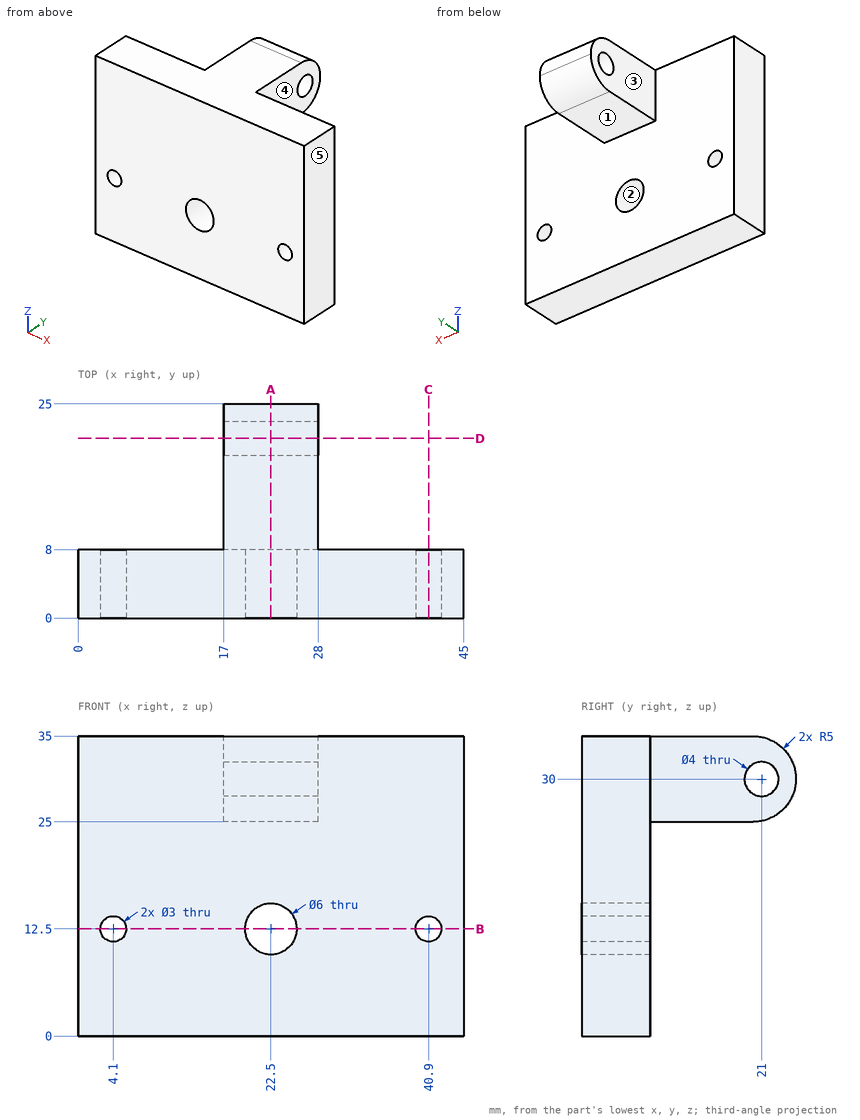
Check sheet for the drawn part. Datum: minimum x, y, z corner. Units: mm. A direction names the side the tool comes from. Round coordinates to 2 decimals unless told otherwise and drop trailing zeros. Order: outer loops, then holes, each group sorted by start corner. A loop starts at its lowest first (then second) coordinate and runs counter-clockwise, first axis right, second up.
1) Section check A-A (x = 22.5). Give the number of separate pieces and of enclosed holes in the cut face, and give its area (3 significant figures).
2) Mould release check, pull along X, two halves, no side actions. Record for the marked faces 1, 2 and 3: +X half, -X half, draft (parallel to the pull), parting line (faces both ways), or undercut.
3) Section check C-C (x = 40.9). Record the boundary of the cut face in (y, z), and give its area (3 significant figures).
4) Go/stop test with flat-tipped pins: pin 1 Ø4 at (x, z) = (40.9, 12.5) entering from +Y; pin 2 Ø4 at (y, z) = (10.5, 28.5) entering from -X; pin 3 Ø3 at (y, z) = (21, 30) entering from +X; pin 4 Ø3.5 at (x, y) = (23.5, 12) entering from -Z. Record where each tip stops, or that it passes through.
5) Tool access check on the marked faces 4 and 5. Record the directions out of +Z, -Z, +X, -X, +Y, -Y that give a thin tool (end or side, any length) a straight path to the whole face; none if there is none.
6) Section check B-B (z = 12.5). Record the boundary of the cut face in (x, y), and give its area (3 significant figures).
7) Section check D-D (y = 21). Record the boundary of the cut face in (x, z), and give its area (3 significant figures).
8) Scan lines: line 1 (X direction, y = 4, z = 12.5); line 2 (Y direction, x = 23, z = 30); line 3 (Y direction, x = 27.5, z = 24). Record each from-to range of solid material in increasing order.
Result:
1. separate pieces: 2
1. enclosed holes: 1
1. area: 379 mm2
2. face 1: draft
2. face 2: undercut
2. face 3: -X half
3. outline: (0, 0) - (8, 0) - (8, 11) - (0, 11) - close; (0, 14) - (8, 14) - (8, 35) - (0, 35) - close
3. area: 256 mm2
4. pin 1: stops at y = 8
4. pin 2: stops at x = 17
4. pin 3: passes through
4. pin 4: stops at z = 25
5. face 4: +Z, -Z, +X, +Y
5. face 5: +Z, -Z, +X, +Y, -Y
6. outline: (0, 0) - (2.6, 0) - (2.6, 8) - (0, 8) - close; (5.6, 0) - (19.5, 0) - (19.5, 8) - (5.6, 8) - close; (25.5, 0) - (39.4, 0) - (39.4, 8) - (25.5, 8) - close; (42.4, 0) - (45, 0) - (45, 8) - (42.4, 8) - close
6. area: 264 mm2
7. outline: (17, 25.1) - (28, 25.1) - (28, 28) - (17, 28) - close; (17, 32) - (28, 32) - (28, 34.9) - (17, 34.9) - close
7. area: 63.8 mm2
8. line 1: x = 0 to 2.6, 5.6 to 19.5, 25.5 to 39.4, 42.4 to 45
8. line 2: y = 0 to 19, 23 to 25
8. line 3: y = 0 to 8
